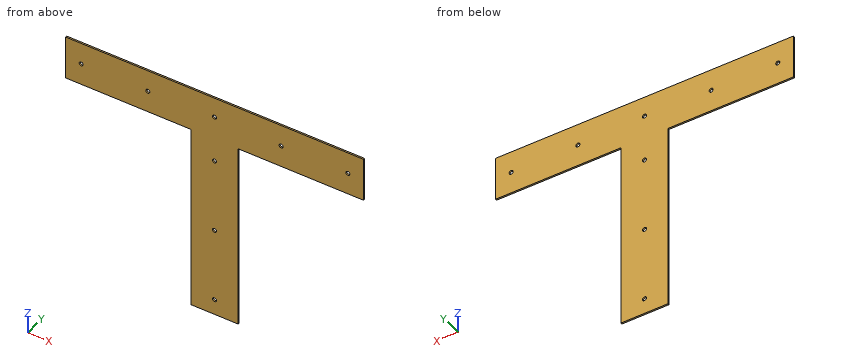
```python
from build123d import *

# Parameters (mm, degrees)
F0_R     = 6.5
F1_DEPTH = 5


with BuildPart() as f1:
    # F0 (on Front) → F1 (new body)
    with BuildSketch(Plane.XZ):
        Polygon((-321.046383, 156.913972), (-321.046383, -443.086028), (-171.046383, -443.086028), (-171.046383, 156.913972), (228.953617, 156.913972), (228.953617, 296.913972), (-721.046383, 296.913972), (-721.046383, 156.913972), align=None)
        with Locations((-246.046383, -393.086028)):
            Circle(F0_R, mode=Mode.SUBTRACT)
        with Locations((-246.046383, -155.586028)):
            Circle(F0_R, mode=Mode.SUBTRACT)
        with Locations((-671.046383, 226.913972)):
            Circle(F0_R, mode=Mode.SUBTRACT)
        with Locations((-458.546383, 226.913972)):
            Circle(F0_R, mode=Mode.SUBTRACT)
        with Locations((-246.046383, 81.913972)):
            Circle(F0_R, mode=Mode.SUBTRACT)
        with Locations((-246.046383, 231.913972)):
            Circle(F0_R, mode=Mode.SUBTRACT)
        with Locations((-33.546383, 226.913972)):
            Circle(F0_R, mode=Mode.SUBTRACT)
        with Locations((178.953617, 226.913972)):
            Circle(F0_R, mode=Mode.SUBTRACT)
    extrude(amount=F1_DEPTH)


solid = f1.part
```
The listing builds one solid part. Answer for the finished solid, in the listing's coordinates (mm). Coordinates: 2 decimals unless noted, no trailing zeros. Loops run counter-clockwise (first coordinate to the right, second up) from the corner with the lowest first, then second, coordinate; pieces in that order, holes last. Notation, with made-up numbers: M 28.5,41.5 L 58.5,41.5 A17 cw 58.5,50.5 Z; hole C 51,-34.5 d1. An arc over 180 degrees is marked long. Answer as CSV lines item,"result". Start each with the question number.
(1) The part is cut by section C-C (x = -94). Give the vertices of the cut face in (y, z).
(2) The part is cut by section B-B (z = -289.5). Give the vertices of the cut face in (x, y), and give its area (3 significant figures).
(3) Find the intervals of material crossed by L1, parallel to X at y = -3.75, z = 136; L2, parallel to Z at x = -345.5, y = -2, in increasing order. Write a range as [from, to].
(4) The part is cut by section A-A (y = -3.2). State how many separate pieces and enclosed holes the cut face has, and give its area (3 significant figures).
(5) Given pin 1 (1.5 mm diameter, centred on x = -152.5, y = -1, fed in from -Z); pin 2 (21 mm diameter, centred on x = -246.05, z = 231.91, fed in from +Y); pin 3 (2.5 mm diameter, centred on y = -1.5, z = -96, fed in from -X); pin 4 (2.5 mm diameter, centred on y = -3, z = -99, fed in from +X), each flat-ended and moving along its own axis, determine where each tip first touches the part or whether it passes through.
Determined:
1,outline,"M -5,156.91 L 0,156.91 L 0,296.91 L -5,296.91 Z"
2,outline,"M -321.05,-5 L -171.05,-5 L -171.05,0 L -321.05,0 Z"
2,area,"750 mm2"
3,L1,"[-321.05, -171.05]"
3,L2,"[156.91, 296.91]"
4,separate pieces,"1"
4,enclosed holes,"8"
4,area,"222,000 mm2"
5,pin 1,"z = 156.91"
5,pin 2,"y = 0"
5,pin 3,"x = -321.05"
5,pin 4,"x = -171.05"
